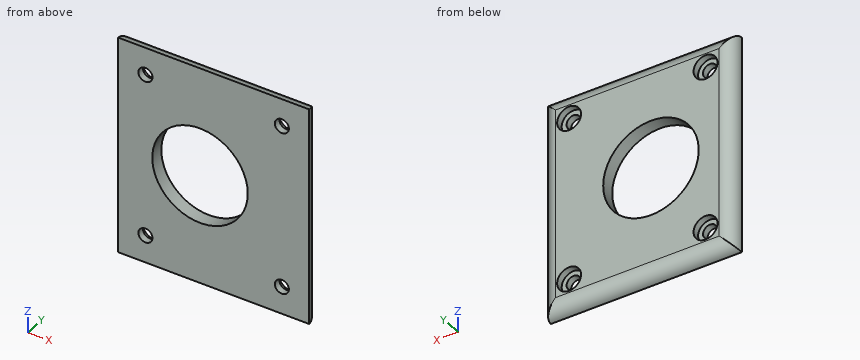
Autodesk Inventor part; units mm, degrees
ref_plane "YZ Plane" through (0, 0, 0) normal (1, 0, 0) x (0, 1, 0)
ref_plane "XZ Plane" through (0, 0, 0) normal (0, 1, 0) x (-1, 0, 0)
ref_plane "XY Plane" through (0, 0, 0) normal (0, 0, 1) x (1, 0, 0)
sketch "Sketch1" plane through (0, 0, 0) normal (0, 1, 0) x (-1, 0, 0)
  line L0 (0, 0) -> (44.45, 0)
  line L1 (44.45, 0) -> (44.45, -50.4952)
  line L2 (44.45, -50.4952) -> (0, -50.4952)
  line L3 (0, -50.4952) -> (0, 0)
  dimension "d0" = 44.45
  dimension "d1" = 50.4952
extrude "Extrusion1" add sketch "Sketch1" along normal blind 3.175
sketch "Sketch2" plane through (0, 3.175, 0) normal (0, 1, 0) x (1, 0, 0)
  line L0 (-44.45, 50.4952) -> (-44.45, 0)
  line L1 (-44.45, 50.4952) -> (-38.1, 50.4952)
  line L2 (0, 50.4952) -> (-44.45, 50.4952)
  line L3 (-38.1, 50.4952) -> (-38.1, 44.1452)
  line L4 (-44.45, 0) -> (0, 0)
  line L5 (0, 0) -> (-6.35, 0)
  line L6 (-6.35, 0) -> (-6.35, 6.35)
  line L7 (-44.45, 50.4952) -> (-44.45, 25.2476)
  line L8 (-44.45, 25.2476) -> (-25.4, 25.2476)
  circle A0 centre (-25.4, 25.2476) radius 11.1125
  line L9 (-44.45, 0) -> (-38.1, 0)
  line L10 (-38.1, 0) -> (-38.1, 6.35)
  line L11 (0, 0) -> (0, 50.4952)
  line L12 (0, 50.4952) -> (-6.35, 50.4952)
  line L13 (-6.35, 44.1452) -> (-6.35, 50.4952)
  dimension "d4" = 6.35
  dimension "d5" = 6.35
  dimension "d6" = 6.35
  dimension "d7" = 6.35
  dimension "d15" = 25.2476
  dimension "d16" = 19.05
  dimension "d17" = 22.225
  dimension "d21" = 6.35
  dimension "d22" = 6.35
  dimension "d23" = 6.35
hole "Hole1" at (-6.35, 3.175, -6.35) at (-38.1, 3.175, -44.1452) at (-6.35, 3.175, -44.1452) at (-38.1, 3.175, -6.35) direction (0, -1, 0) diameter 3.2766 depth 12.7 tip angle 118 counterbore diameter 5.5626 counterbore depth 1.5875
extrude "Extrusion2" cut sketch "Sketch2" against normal blind 3.175 contours A0
fillet "Fillet1" radius 3.175 4 edges at (-44.45, 3.175, -25.2476) (-22.225, 3.175, -50.4952) (0, 3.175, -25.2476) (-22.225, 3.175, 0)
properties part number "sample holder lid for neutron r2"
For this review, take the finished solid that the model builds, in its own axes (mm). Round coordinates to 2 decimals unless told otherwise and drop trailing zeros. One line per item, written item: value. Start each with the question number.
Item 1: Clearance check with flat-ended pins moving along their axes: pin 1 Ø1 at (x, y) = (-15, 2) entering from +Z; pin 2 Ø5 at (x, z) = (-38.1, -44.15) entering from +Y; pin 3 Ø1 at (x, y) = (-20, 1.5) entering from +Z. State where each tip first meets the part, or that it passes through.
Item 2: Take a section at A-A (z = -6.35). State how many separate pieces and enclosed holes the cut face has, plus the area to 3 significant figures.
Item 3: For L1, parallel to Z at x = -6.35, y = 0.45; L2, parallel to Z at x = -6.35, y = 2.8; L3, parallel to Z at x = -21, y = 1.4, list the stretches that pass through material, from the lowest coordinate up.
Answer below:
1. pin 1: stops at z = -0.38
1. pin 2: stops at y = 1.59
1. pin 3: stops at z = -0.16
2. separate pieces: 3
2. enclosed holes: 0
2. area: 109 mm2
3. L1: z = -50.46 to -45.78, -42.51 to -7.99, -4.71 to -0.03
3. L2: z = -48.82 to -46.93, -41.36 to -9.13, -3.57 to -1.68
3. L3: z = -50.17 to -35.45, -15.04 to -0.33
